from build123d import *

# Parameters (mm, degrees)
F1_DEPTH  = 10
F2_DEPTH  = 25
F3_DEPTH  = 25
F4_DEPTH  = 25
F5_DEPTH  = 25
F6_DEPTH  = 25
F7_DEPTH  = 25
F8_DEPTH  = 25
F9_DEPTH  = 25
F10_DEPTH = 25
F11_DEPTH = 25
F12_DEPTH = 25
F13_DEPTH = 25
F14_DEPTH = 25
F15_DEPTH = 25
F16_DEPTH = 25
F17_SIZE  = 5
F0_R      = 10
F18_DEPTH = 5


with BuildPart() as f1:
    # F0 (on Top) → F1 (new body)
    with BuildSketch(Plane.XY):
        Polygon((-96.6750791953, 70.3877321793), (-109.1969291758, 48.7497121768), (-116.9463493664, 24.9810958252), (-119.5846529188, 0.1206857134), (-116.9965333079, -24.7449989432), (-109.2951037797, -48.5292084063), (-96.8169537602, -70.1924585931), (-80.1074382822, -88.7879615186), (-59.8968433531, -103.5030044738), (-37.0684689525, -113.6944694709), (-12.6200245844, -118.9169405856), (12.3799754156, -118.9421707699), (36.8389110842, -113.7690573437), (59.6878095658, -103.6236901871), (79.9280643554, -88.9494705277), (96.6750791953, -70.3877321793), (109.1969291758, -48.7497121768), (116.9463493664, -24.9810958252), (119.5846529188, -0.1206857134), (116.9965333079, 24.7449989432), (109.2951037797, 48.5292084063), (96.8169537602, 70.1924585931), (80.1074382822, 88.7879615186), (59.8968433531, 103.5030044738), (37.0684689525, 113.6944694709), (12.6200245844, 118.9169405856), (-12.3799754156, 118.9421707699), (-36.8389110842, 113.7690573437), (-59.6878095658, 103.6236901871), (-79.9280643554, 88.9494705277), align=None)
        Polygon((-8.6753877305, -14.9912523735), (-17.3204992552, 0.0174799755), (-8.6451115247, 15.008732349), (8.6753877305, 14.9912523735), (17.3204992552, -0.0174799755), (8.6451115247, -15.008732349), align=None, mode=Mode.SUBTRACT)
    extrude(amount=F1_DEPTH)

    # F2 (add): a face of the model
    f2_faces = [f1.faces().sort_by_distance(p)[0] for p in [
        (0.1200245844, 118.9295556778, 5),
    ]]
    extrude(f2_faces, amount=F2_DEPTH)

    # F3 (add): a face of the model
    f3_faces = [f1.faces().sort_by_distance(p)[0] for p in [
        (-48.263360325, 108.6963737654, 5),
    ]]
    extrude(f3_faces, amount=F3_DEPTH)

    # F4 (add): a face of the model
    f4_faces = [f1.faces().sort_by_distance(p)[0] for p in [
        (-88.3015717753, 79.6686013535, 5),
    ]]
    extrude(f4_faces, amount=F4_DEPTH)

    # F5 (add): a face of the model
    f5_faces = [f1.faces().sort_by_distance(p)[0] for p in [
        (-113.0716392711, 36.865404001, 5),
    ]]
    extrude(f5_faces, amount=F5_DEPTH)

    # F6 (add): a face of the model
    f6_faces = [f1.faces().sort_by_distance(p)[0] for p in [
        (-118.2905931133, -12.3121566149, 5),
    ]]
    extrude(f6_faces, amount=F6_DEPTH)

    # F7 (add): a face of the model
    f7_faces = [f1.faces().sort_by_distance(p)[0] for p in [
        (48.4826561528, 108.5987369723, 5),
    ]]
    extrude(f7_faces, amount=F7_DEPTH)

    # F8 (add): a face of the model
    f8_faces = [f1.faces().sort_by_distance(p)[0] for p in [
        (88.4621960212, 79.4902100558, 5),
    ]]
    extrude(f8_faces, amount=F8_DEPTH)

    # F9 (add): a face of the model
    f9_faces = [f1.faces().sort_by_distance(p)[0] for p in [
        (113.1458185438, 36.6371036748, 5),
    ]]
    extrude(f9_faces, amount=F9_DEPTH)

    # F10 (add): a face of the model
    f10_faces = [f1.faces().sort_by_distance(p)[0] for p in [
        (118.2655011426, -12.5508907693, 5),
    ]]
    extrude(f10_faces, amount=F10_DEPTH)

    # F11 (add): a face of the model
    f11_faces = [f1.faces().sort_by_distance(p)[0] for p in [
        (102.9360041856, -59.5687221781, 5),
    ]]
    extrude(f11_faces, amount=F11_DEPTH)

    # F12 (add): a face of the model
    f12_faces = [f1.faces().sort_by_distance(p)[0] for p in [
        (69.8079369606, -96.2865803574, 5),
    ]]
    extrude(f12_faces, amount=F12_DEPTH)

    # F13 (add): a face of the model
    f13_faces = [f1.faces().sort_by_distance(p)[0] for p in [
        (24.6094432499, -116.3556140568, 5),
    ]]
    extrude(f13_faces, amount=F13_DEPTH)

    # F14 (add): a face of the model
    f14_faces = [f1.faces().sort_by_distance(p)[0] for p in [
        (-24.8442467684, -116.3057050283, 5),
    ]]
    extrude(f14_faces, amount=F14_DEPTH)

    # F15 (add): a face of the model
    f15_faces = [f1.faces().sort_by_distance(p)[0] for p in [
        (-70.0021408176, -96.1454829962, 5),
    ]]
    extrude(f15_faces, amount=F15_DEPTH)

    # F16 (add): a face of the model
    f16_faces = [f1.faces().sort_by_distance(p)[0] for p in [
        (-103.05602877, -59.3608334997, 5),
    ]]
    extrude(f16_faces, amount=F16_DEPTH)

    # F17
    f17_edges = [f1.edges().sort_by_distance(p)[0] for p in [
        (144.44505, -2.758988, 5),
        (141.806747, -27.619398, 5),
        (140.780731, 32.446425, 5),
        (133.079301, 56.230634, 5),
        (115.412447, 86.901966, 5),
        (98.702932, 105.497468, 5),
        (70.088303, 126.331367, 5),
        (47.259929, 136.522832, 5),
        (12.645255, 143.916928, 5),
        (-12.354745, 143.942158, 5),
        (-46.984273, 136.617944, 5),
        (-69.833172, 126.472577, 5),
        (42.012022, -138.227981, 5),
        (17.553086, -143.401094, 5),
        (74.362022, -123.863935, 5),
        (94.602277, -109.189715, 5),
        (-98.489793, 105.696477, 5),
        (-74.611879, -123.713589, 5),
        (-17.842493, -143.365373, 5),
        (-42.290937, -138.142901, 5),
        (-118.480193, -82.670602, 5),
        (-141.862205, -27.333117, 5),
        (-140.714954, 32.730512, 5),
        (-144.450325, -2.467433, 5),
        (-130.958343, -61.007352, 5),
        (-132.965533, 56.499128, 5),
        (-115.236808, 87.134738, 5),
        (130.834938, -61.271556, 5),
        (118.313088, -82.909576, 5),
        (-94.822474, -108.998546, 5),
    ]]
    chamfer(f17_edges, length=F17_SIZE)

    # F0 (on Top) → F18 (join)
    with BuildSketch(Plane.XY):
        Polygon((-96.6750791953, 70.3877321793), (-109.1969291758, 48.7497121768), (-116.9463493664, 24.9810958252), (-119.5846529188, 0.1206857134), (-116.9965333079, -24.7449989432), (-109.2951037797, -48.5292084063), (-96.8169537602, -70.1924585931), (-80.1074382822, -88.7879615186), (-59.8968433531, -103.5030044738), (-37.0684689525, -113.6944694709), (-12.6200245844, -118.9169405856), (12.3799754156, -118.9421707699), (36.8389110842, -113.7690573437), (59.6878095658, -103.6236901871), (79.9280643554, -88.9494705277), (96.6750791953, -70.3877321793), (109.1969291758, -48.7497121768), (116.9463493664, -24.9810958252), (119.5846529188, -0.1206857134), (116.9965333079, 24.7449989432), (109.2951037797, 48.5292084063), (96.8169537602, 70.1924585931), (80.1074382822, 88.7879615186), (59.8968433531, 103.5030044738), (37.0684689525, 113.6944694709), (12.6200245844, 118.9169405856), (-12.3799754156, 118.9421707699), (-36.8389110842, 113.7690573437), (-59.6878095658, 103.6236901871), (-79.9280643554, 88.9494705277), align=None)
        Polygon((-8.6753877305, -14.9912523735), (-17.3204992552, 0.0174799755), (-8.6451115247, 15.008732349), (8.6753877305, 14.9912523735), (17.3204992552, -0.0174799755), (8.6451115247, -15.008732349), align=None, mode=Mode.SUBTRACT)
        Polygon((-8.6451115247, 15.008732349), (-17.3204992552, 0.0174799755), (-8.6753877305, -14.9912523735), (8.6451115247, -15.008732349), (17.3204992552, -0.0174799755), (8.6753877305, 14.9912523735), align=None)
        Circle(F0_R, mode=Mode.SUBTRACT)
    extrude(amount=F18_DEPTH)


solid = f1.part
Design review of the part built by this model. Coordinates are the model's own, in mm. A direction names the side the tool comes from. Coordinates: 2 decimals unless noted, no trailing zeros. Loops run counter-clockwise (first coordinate to the right, second up) from the corner with the lowest first, then second, coordinate; pieces in that order, holes last. Notation, with made-up numbers: (41, 33.25) -> (72, 33.25) arc R15 ccw to (72, 62.25) -> close; hole circle Ø1 at (-31.5, -31). An arc over 180 degrees is marked (long way). Use a Markdown table: item, result. Add a question column.
Item 1: We need section B-B, the plane y = -84. Write out the cut boundary in (x, z).
Item 2: Wall thickness on L1, parallel to X at y = -75, z = 8; L2, parallel to X at y = 119, z = 7.5; L3, parallel to Y at x = 0, z = 2.9: over which ranges is each line inside the solid? List them lowest first. Write a range as from..to.
Item 3: Clearance check with flat-ended pins moving along their axes: P1, Ø6, axis at y = -95, z = 7, coming from the +X side; P2, Ø9, axis at x = 7, y = -4.5, coming from the +Z side; P3, Ø6, axis at x = 46.5, z = 5, coming from the +Y side. State where each tip first meets the part, or that it passes through.
Item 4: Machinability: for faces 1 (the flat face through (-48.301, 133.336, 4.93)), 2 (the flat face through (118.31, 12.14, 4.93)), 3 (the flat face through (126.75, -26.02, 4.93)), 4 (the flat face through (65.48, -111.61, 4.93)), 5 (the flat face through (-127.557, -61.974, 4.93)), which of the approach directions +Z, -Z, +X, -X, +Y, -Y give a long, thin tool a straight path to every point of the face, cutting with its end or side? Answer none if there is none.
Item 5: We need section A-A, the plane x = 0. Write out the cut boundary in (y, z).
Item 6: The part is to be moulded in two halves that separate along Y. For faces 6 (the flat face through (-106.793, 96.494, 4.93)), 7 (the flat face through (-39.13, -123.34, 4.93)), 8 (the flat face through (29.68, -140.836, 4.93)), say which applies: +Y half, -Y half, draft (parallel to the pull), parting line (faces both ways), or undercut.
Numbers:
| question | item | result |
|---|---|---|
| 1 | outline | (-84.41, 0) -> (84.39, 0) -> (84.39, 10) -> (-84.41, 10) -> close |
| 2 | L1 | x = -122.9..-105.16, -92.5..92.51, 104.65..122.89 |
| 2 | L2 | x = -66.52..-39.16, -12.38..12.62, 39.44..66.82 |
| 2 | L3 | y = -118.93..-10, 10..143.93 |
| 3 | P1 | stops at x = 86.49 |
| 3 | P2 | stops at z = 5 |
| 3 | P3 | stops at y = 133.59 |
| 4 | face 1 | +Z, -Z, +Y |
| 4 | face 2 | +Z, -Z, +X |
| 4 | face 3 | +Z, -Z |
| 4 | face 4 | +Z, -Z, -Y |
| 4 | face 5 | +Z, -Z, -X |
| 5 | outline | (-118.93, 0) -> (-10, 0) -> (-10, 5) -> (-15, 5) -> (-15, 10) -> (-118.93, 10) -> close; (10, 0) -> (143.93, 0) -> (143.93, 10) -> (15, 10) -> (15, 5) -> (10, 5) -> close |
| 6 | face 6 | +Y half |
| 6 | face 7 | undercut |
| 6 | face 8 | -Y half |
